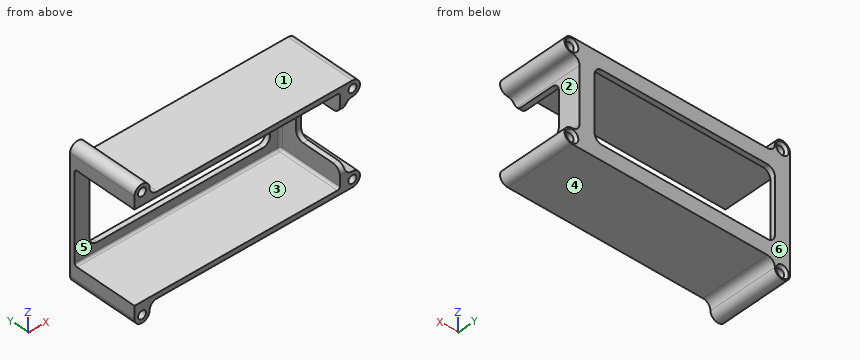
from build123d import *

# Parameters (mm, degrees)
SKETCH1_W           = 133.35
SKETCH1_H           = 63.5
SKETCH1_W_2         = 127
SKETCH1_H_2         = 57.15
BOSS_EXTRUDE1_DEPTH = 41.275
SKETCH2_W           = 31.75
SKETCH2_H           = 60.325
CUT_EXTRUDE1_DEPTH  = 134.35
SKETCH3_W           = 133.35
SKETCH3_H           = 63.5
SKETCH3_W_2         = 114.3
SKETCH3_H_2         = 44.45
BOSS_EXTRUDE2_DEPTH = 3.175
BOSS_EXTRUDE3_DEPTH = 44.45
SKETCH6_R           = 2.54
BOSS_EXTRUDE4_DEPTH = 44.45
CUT_EXTRUDE2_DEPTH  = 4.175
FILLET1_R           = 1.5875
FILLET2_R           = 4.7625


with BuildPart() as part:
    # Sketch1 → Boss-Extrude1 (new body)
    with BuildSketch(Plane(origin=(0, 0, 0), x_dir=(1, 0, 0), z_dir=(0, 1, 0))):
        Rectangle(SKETCH1_W, SKETCH1_H)
        Rectangle(SKETCH1_W_2, SKETCH1_H_2, mode=Mode.SUBTRACT)
    extrude(amount=BOSS_EXTRUDE1_DEPTH)

    # Sketch2 → Cut-Extrude1 (cut, through all)
    with BuildSketch(Plane.ZY.offset(66.675)):
        Rectangle(SKETCH2_W, SKETCH2_H)
    extrude(amount=-CUT_EXTRUDE1_DEPTH, mode=Mode.SUBTRACT)

    # Sketch3 → Boss-Extrude2 (add)
    with BuildSketch(Plane(origin=(0, 41.275, 0), x_dir=(1, 0, 0), z_dir=(0, 1, 0))):
        Rectangle(SKETCH3_W, SKETCH3_H)
        Rectangle(SKETCH3_W_2, SKETCH3_H_2, mode=Mode.SUBTRACT)
    extrude(amount=BOSS_EXTRUDE2_DEPTH)

    # Sketch4 → Boss-Extrude3 (add)
    with BuildSketch(Plane(origin=(0, 44.45, 0), x_dir=(1, 0, 0), z_dir=(0, 1, 0))):
        with BuildLine():
            Line((71.4375, 31.75), (66.675, 31.75))
            Line((66.675, 31.75), (66.675, 17.4625))
            ThreePointArc((66.675, 17.4625), (68.069903955, 20.830096045), (71.4375, 22.225))
            ThreePointArc((71.4375, 22.225), (76.2, 26.9875), (71.4375, 31.75))
        make_face()
    boss_extrude3 = extrude(amount=-BOSS_EXTRUDE3_DEPTH)

    # Sketch5 → Cut-Revolve1 (revolve, cut)
    with BuildSketch(Plane.YZ.offset(71.4375)):
        Polygon((0, -29.5275), (42.8625, -29.5275), (44.45, -30.982175739), (44.45, -26.9875), (0, -26.9875), align=None)
    cut_revolve1 = revolve(axis=Axis((71.4375, 44.45, -26.9875), (0, -1, 0)), mode=Mode.SUBTRACT)

    # Sketch6 → Boss-Extrude4 (add)
    with BuildSketch(Plane(origin=(0, 44.45, 0), x_dir=(1, 0, 0), z_dir=(0, 1, 0))):
        with BuildLine():
            Line((-66.675, 36.5125), (-66.675, 31.75))
            Line((-66.675, 31.75), (-52.3875, 31.75))
            ThreePointArc((-52.3875, 31.75), (-55.755096045, 33.144903955), (-57.15, 36.5125))
            ThreePointArc((-57.15, 36.5125), (-61.9125, 41.275), (-66.675, 36.5125))
        make_face()
        with Locations((-61.9125, 36.5125)):
            Circle(SKETCH6_R, mode=Mode.SUBTRACT)
    boss_extrude4 = extrude(amount=-BOSS_EXTRUDE4_DEPTH)

    # Sketch7 → Cut-Revolve2 (revolve, cut)
    with BuildSketch(Plane(origin=(-61.9125, 0, 0), x_dir=(0, 1, 0), z_dir=(-1, 0, 0))):
        Polygon((42.8625, 39.0525), (44.45, 40.507175739), (44.45, 36.5125), (42.8625, 36.5125), align=None)
    cut_revolve2 = revolve(axis=Axis((-61.9125, 42.8625, -36.5125), (0, -1, 0)), mode=Mode.SUBTRACT)

    # Mirror1: Boss-Extrude3, Cut-Revolve1, Boss-Extrude4, Cut-Revolve2 across plane
    add(boss_extrude3.mirror(Plane.XY))
    add(cut_revolve1.mirror(Plane.XY), mode=Mode.SUBTRACT)
    add(boss_extrude4.mirror(Plane.XY))
    add(cut_revolve2.mirror(Plane.XY), mode=Mode.SUBTRACT)

    # Sketch8 → Cut-Extrude2 (cut, through all)
    with BuildSketch(Plane(origin=(-63.5, 0, 0), x_dir=(0, 0, -1), z_dir=(1, 0, 0))):
        Polygon((-15.875, 0), (-15.875, 30.1625), (15.875, 30.1625), (15.875, 0), (28.575, 0), (28.575, 41.275), (-28.575, 41.275), (-28.575, 0), align=None)
    extrude(amount=-CUT_EXTRUDE2_DEPTH, mode=Mode.SUBTRACT)

    # Fillet1
    fillet1_edges = [part.edges().sort_by_distance(p)[0] for p in [
        (63.5, 20.6375, 28.575),
        (63.5, 20.6375, -28.575),
        (63.5, 41.275, 0),
        (-1.5875, 41.275, -28.575),
        (-1.5875, 41.275, 28.575),
    ]]
    fillet(fillet1_edges, radius=FILLET1_R)

    # Fillet2
    fillet2_edges = [part.edges().sort_by_distance(p)[0] for p in [
        (65.0875, 0, 15.875),
        (65.0875, 30.1625, 15.875),
        (65.0875, 0, -15.875),
        (65.0875, 30.1625, -15.875),
        (-57.15, 42.8625, 22.225),
        (57.15, 42.8625, 22.225),
        (57.15, 42.8625, -22.225),
        (-57.15, 42.8625, -22.225),
    ]]
    fillet(fillet2_edges, radius=FILLET2_R)


solid = part.part
Can you work these out from the model? Positions are in its coordinate system, mm. Face numbers are marked on the shaded views. A direction names the side the tool comes from. Coordinates: 2 decimals unless noted, no trailing zeros. Return JSON: item names as keys, results as strings. Group by question number.
Item 1: We'd pull the mould along Z, two halves only. Please class the marked faces 1, 2, 3 and 4: pulls with the +Z half, pulls with the -Z half, needs draft (parallel to the pull), parting line crosses it, or undercut.
Item 2: I'm going to push flat-ended pins straight in: pin 1 Ø10 at (x, y) = (25, 35.5) entering from -Z; pin 2 Ø2 at (x, y) = (36.5, 8) entering from +Z; pin 3 Ø3.5 at (y, z) = (42.5, 2) entering from +X (3 decimals). Where does each tip first touch, or does it pass through?
Item 3: Which directions (+Z, -Z, +X, -X, +Y, -Y) give clear straight access to the entire face, cutting with the end or side of a thin tool? Please do the marked faces 5 and 6.
Item 4: Please list where these lines run through material, in increasing order: probe 1 along Z at (x, y) = (13, 23) (3 decimals); probe 2 along X at (y, z) = (5, 27); probe 3 along Y at (x, z) = (25.5, -23.5) (3 decimals).
Item 5: If we section it at A-A (y = 21): Count the separate pieces of the cut face and the enclosed holes in it, then the cut area to 3 significant figures.
Return value:
{
 "1": {"face 1": "pulls with the +Z half", "face 2": "undercut", "face 3": "undercut", "face 4": "pulls with the -Z half"},
 "2": {"pin 1": "stops at z = -31.75", "pin 2": "stops at z = 31.75", "pin 3": "stops at x = 66.675"},
 "3": {"face 5": "-X, -Y", "face 6": "+Z, -Z, +X, -X, +Y"},
 "4": {"probe 1": "z = -31.75 to -28.575, 28.575 to 31.75", "probe 2": "x = 63.5 to 68.9, 73.98 to 76.2", "probe 3": "y = 41.275 to 44.45"},
 "5": {"separate pieces": "2", "enclosed holes": "4", "area": "1,190 mm^2"}
}
